```python
from build123d import *

# Parameters (mm, degrees)
SKETCH1_R           = 4.572
SKETCH1_R_2         = 1.75
BOSS_EXTRUDE1_DEPTH = 3.2004
BOSS_EXTRUDE2_START = -3.429
SKETCH1_3_R         = 1.75
BOSS_EXTRUDE2_DEPTH = 3.429


with BuildPart() as part:
    # Sketch1 → Boss-Extrude1 (new body)
    with BuildSketch(Plane(origin=(0, 0, 0), x_dir=(1, 0, 0), z_dir=(0, 1, 0))):
        with BuildLine():
            Line((15.494618326, -9.079673628), (9.632116129, 0))
            Line((9.632116129, 0), (20.267125172, 16.471194022))
            ThreePointArc((20.267125172, 16.471194022), (19.901971998, 19.901971998), (16.471194022, 20.267125172))
            Line((16.471194022, 20.267125172), (0, 9.632116129))
            Line((0, 9.632116129), (-9.079673628, 15.494618326))
            ThreePointArc((-9.079673628, 15.494618326), (-14.877526676, 14.877526676), (-15.494618326, 9.079673628))
            Line((-15.494618326, 9.079673628), (-9.632116129, 0))
            Line((-9.632116129, 0), (-15.494618326, -9.079673628))
            ThreePointArc((-15.494618326, -9.079673628), (-14.877526676, -14.877526676), (-9.079673628, -15.494618326))
            Line((-9.079673628, -15.494618326), (0, -9.632116129))
            Line((0, -9.632116129), (9.079673628, -15.494618326))
            ThreePointArc((9.079673628, -15.494618326), (14.877526676, -14.877526676), (15.494618326, -9.079673628))
        make_face()
        with Locations(Location((0, 0, 0), (0, 0, 270))):
            Circle(SKETCH1_R, mode=Mode.SUBTRACT)
        with Locations(Location((17.960512242, 17.960512242, 0), (0, 0, 270))):
            Circle(SKETCH1_R_2, mode=Mode.SUBTRACT)
    extrude(amount=BOSS_EXTRUDE1_DEPTH)

    # Sketch1_3 → Boss-Extrude2 (add)
    with BuildSketch(Plane(origin=(0, 0, 0), x_dir=(1, 0, 0), z_dir=(0, 1, 0)).offset(BOSS_EXTRUDE2_START)):
        with BuildLine():
            ThreePointArc((16.471194022, 20.267125172), (19.901971998, 19.901971998), (20.267125172, 16.471194022))
            Line((20.267125172, 16.471194022), (15.494618326, 9.079673628))
            Line((15.494618326, 9.079673628), (9.632116129, 0))
            Line((9.632116129, 0), (15.494618326, -9.079673628))
            ThreePointArc((15.494618326, -9.079673628), (14.877526676, -14.877526676), (9.079673628, -15.494618326))
            Line((9.079673628, -15.494618326), (0, -9.632116129))
            Line((0, -9.632116129), (-9.079673628, -15.494618326))
            ThreePointArc((-9.079673628, -15.494618326), (-14.877526676, -14.877526676), (-15.494618326, -9.079673628))
            Line((-15.494618326, -9.079673628), (-9.632116129, 0))
            Line((-9.632116129, 0), (-15.494618326, 9.079673628))
            ThreePointArc((-15.494618326, 9.079673628), (-14.877526676, 14.877526676), (-9.079673628, 15.494618326))
            Line((-9.079673628, 15.494618326), (0, 9.632116129))
            Line((0, 9.632116129), (9.079673628, 15.494618326))
            Line((9.079673628, 15.494618326), (16.471194022, 20.267125172))
        make_face()
        with Locations(Location((17.960512242, 17.960512242, 0), (0, 0, 270))):
            Circle(SKETCH1_3_R, mode=Mode.SUBTRACT)
        with BuildLine():
            Line((8.023816422, 1.021082558), (13.894226547, 10.113003756))
            ThreePointArc((13.894226547, 10.113003756), (13.530488258, 13.530488258), (10.113003756, 13.894226547))
            Line((10.113003756, 13.894226547), (1.021082558, 8.023816422))
            ThreePointArc((1.021082558, 8.023816422), (0, 7.408645479), (-1.021082558, 8.023816422))
            Line((-1.021082558, 8.023816422), (-10.113003756, 13.894226547))
            ThreePointArc((-10.113003756, 13.894226547), (-13.530488258, 13.530488258), (-13.894226547, 10.113003756))
            Line((-13.894226547, 10.113003756), (-8.023816422, 1.021082558))
            ThreePointArc((-8.023816422, 1.021082558), (-7.408645479, 0), (-8.023816422, -1.021082558))
            Line((-8.023816422, -1.021082558), (-13.894226547, -10.113003756))
            ThreePointArc((-13.894226547, -10.113003756), (-13.530488258, -13.530488258), (-10.113003756, -13.894226547))
            Line((-10.113003756, -13.894226547), (-1.021082558, -8.023816422))
            ThreePointArc((-1.021082558, -8.023816422), (0, -7.408645479), (1.021082558, -8.023816422))
            Line((1.021082558, -8.023816422), (10.113003756, -13.894226547))
            ThreePointArc((10.113003756, -13.894226547), (13.530488258, -13.530488258), (13.894226547, -10.113003756))
            Line((13.894226547, -10.113003756), (8.023816422, -1.021082558))
            ThreePointArc((8.023816422, -1.021082558), (7.408645479, 0), (8.023816422, 1.021082558))
        make_face(mode=Mode.SUBTRACT)
    extrude(amount=BOSS_EXTRUDE2_DEPTH)


solid = part.part
```
Part model, mm, in its own coordinate system. A direction names the side the tool comes from. Round coordinates to 2 decimals unless told otherwise and drop trailing zeros. Loops run counter-clockwise (first coordinate to the right, second up) from the corner with the lowest first, then second, coordinate; pieces in that order, holes last.
1. Flat gauge pins, fed straight in: pin 1 (2 mm diameter, centred on x = -1.5, y = 1, fed in from -Z); pin 2 (1.5 mm diameter, centred on y = 2.5, z = 4.5, fed in from +X); pin 3 (1.5 mm diameter, centred on x = -7.5, z = 2.5, fed in from -Y). Where does each tip first touch, or does it go through?
Solutions:
pin 1: stops at z = -11.25
pin 2: stops at x = 13.02
pin 3: stops at y = 0
2. Drill centre lines: line 1 along Z through (x, y) = (13, -0.25); line 2 along X through (y, z) = (2.2, 0); line 3 along X through (y, z) = (-2.5, 13). Where is each one in solid material? Low to high.
Solutions:
line 1: z = -18.03 to -13.94, -8.73 to -5.22, 5.22 to 8.73, 13.94 to 16.02
line 2: x = -9.63 to -4.57, 4.57 to 9.63
line 3: x = -16.02 to -13.94, -8.73 to -5.22, 5.22 to 8.73, 13.94 to 16.02
3. Slice it at C-C (z = 11). Give the cut face in (x, y).
Solutions:
outline: (-16.2, -3.43) - (-14.27, -3.43) - (-14.27, 0) - (-5.63, 0) - (-5.63, -3.43) - (-2.12, -3.43) - (-2.12, 3.2) - (-16.2, 3.2) - close; (2.12, -3.43) - (5.63, -3.43) - (5.63, 0) - (14.27, 0) - (14.27, -3.43) - (16.2, -3.43) - (16.2, 3.2) - (2.12, 3.2) - close
4. Slice it at B-B (y = 1.5). Give the cut face in (x, z).
Solutions:
outline: (-15.49, -9.08) arc R4.64 ccw to (-9.08, -15.49) - (0, -9.63) - (16.47, -20.27) arc R2.75 ccw to (20.27, -16.47) - (9.63, 0) - (15.49, 9.08) arc R4.64 ccw to (9.08, 15.49) - (0, 9.63) - (-9.08, 15.49) arc R4.64 ccw to (-15.49, 9.08) - (-9.63, 0) - close; hole circle Ø9.14 at (0, 0); hole circle Ø3.5 at (17.96, -17.96)
5. Slice it at A-A (x = 18.5). Give the cut face in (y, z), and give its area (3 significant figures).
Solutions:
outline: (-3.43, -20.65) - (3.2, -20.65) - (3.2, -19.63) - (-3.43, -19.63) - close; (-3.43, -16.3) - (3.2, -16.3) - (3.2, -13.73) - (-3.43, -13.73) - close
area: 23.8 mm2
6. Slice it at D-D (x = 2). Give the cut face in (y, z), and give its area (3 significant figures).
Solutions:
outline: (-3.43, -10.92) - (3.2, -10.92) - (3.2, -4.11) - (0, -4.11) - (0, -8.66) - (-3.43, -8.66) - close; (-3.43, 8.66) - (0, 8.66) - (0, 4.11) - (3.2, 4.11) - (3.2, 10.92) - (-3.43, 10.92) - close
area: 59.2 mm2
7. Two-plate mould, pull along Z, no slides. Class faces 5 (the face through (14.939, -0.161, 14.815)), 6 (the face through (8.12, -0.161, -14.875)), 7 (the face through (-4.476, -0.161, 12.522)), 8 (the face through (8, -3.429, 0)): pulls with the +Z half, pulls with the -Z half, needs draft (parallel to the pull), parting line crosses it, or undercut.
Solutions:
face 5: undercut
face 6: pulls with the -Z half
face 7: pulls with the +Z half
face 8: needs draft
8. 3-axis set-ups, long thin cutter, end or side, ignore diameter. For faces 1 (the face through (-12.522, -0.161, -4.476)), 2 (the face through (15.024, -0.161, -8.351)), 3 (the face through (-4.6, -0.2, -12.6)), 4 (the face through (5.63, -1.74, -11)): which of +Z, -Z, +X, -X, +Y, -Y reach the whole face in a straight line?
Solutions:
face 1: -X, +Y, -Y
face 2: +X, +Y, -Y
face 3: -Z, +Y, -Y
face 4: -Y
